Source: three-view drawing plus pictorial views. Frame: mm from the lowest corner of the part. A direction names the side the tool comes from. Give positions to 0.01 mm unless a question says otherwise; leave off trailing zeros. Write each loop counter-clockwise with the first axis right and the second up, starting at its lowest first coordinate (ties: lowest second). Pieces come first, ordered by that corner, then holes.
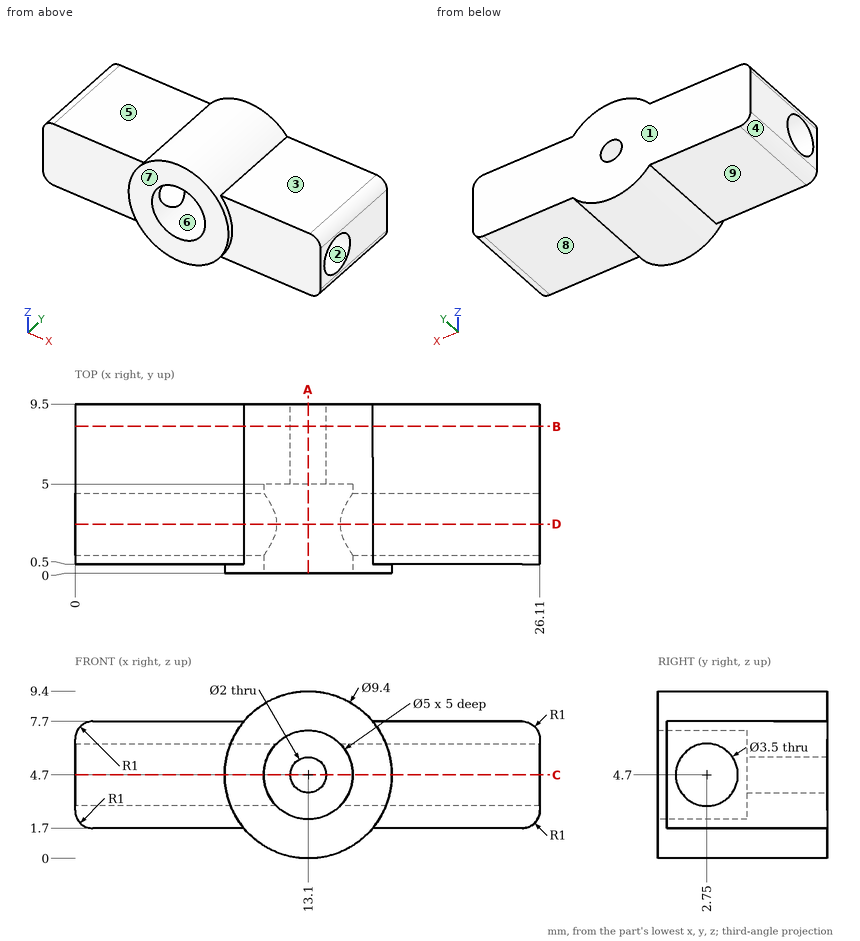
Q1. Section D-D on y = 2.75. Output: boundary loops of the cut face in (x, z), plus the area to 3 significant figures.
Filled sheet:
outline: (0, 2.7) arc R1 ccw to (1, 1.7) - (9.48, 1.7) arc R4.7 ccw to (16.72, 1.7) - (25.11, 1.7) arc R1 ccw to (26.11, 2.7) - (26.11, 2.95) - (14.89, 2.95) arc R2.5 cw to (11.31, 2.95) - (0, 2.95) - close; (0, 6.45) - (11.31, 6.45) arc R2.5 cw to (14.89, 6.45) - (26.11, 6.45) - (26.11, 6.7) arc R1 ccw to (25.11, 7.7) - (16.72, 7.7) arc R4.7 ccw to (9.48, 7.7) - (1, 7.7) arc R1 ccw to (0, 6.7) - close
area: 77.8 mm2
Q2. Ray query, line 1 along Y through (x, z) = (7, 4.7); line 2 along Y through (x, z) = (24.5, 2.5); line 3 along Z through (x, y) = (23.5, 7.5). Return the intervals inside material, ascending.
Filled sheet:
line 1: y = 0.5 to 1, 4.5 to 9.5
line 2: y = 0.5 to 9.5
line 3: z = 1.7 to 7.7
Q3. Pin query (flat end, axial travel): P1, Ø1.8, axis at x = 13.1, z = 4.7, coming from the +Y side; P2, Ø4, axis at x = 23, y = 3, coming from the +Z side; P3, Ø2.5, axis at x = 13, z = 4, coming from the -Y side; P4, Ø1.8, axis at x = 3.5, z = 5.5, coming from the -Y side. Return the tip coordinate at first contact, or that it passes through.
Filled sheet:
P1: passes through
P2: stops at z = 7.7
P3: stops at y = 5
P4: stops at y = 0.5
Q4. Section C-C on z = 4.7. Output: boundary loops of the cut face in (x, y).
Filled sheet:
outline: (0, 0.5) - (8.4, 0.5) - (8.4, 0) - (10.6, 0) - (10.6, 1) - (0, 1) - close; (0, 4.5) - (10.6, 4.5) - (10.6, 5) - (12.1, 5) - (12.1, 9.5) - (0, 9.5) - close; (14.1, 5) - (15.6, 5) - (15.6, 4.5) - (26.11, 4.5) - (26.11, 9.5) - (14.1, 9.5) - close; (15.6, 0) - (17.8, 0) - (17.8, 0.5) - (26.11, 0.5) - (26.11, 1) - (15.6, 1) - close
Q5. Section B-B on y = 8.25. Output: boundary loops of the cut face in (x, z).
Filled sheet:
outline: (0, 2.7) arc R1 ccw to (1, 1.7) - (9.48, 1.7) arc R4.7 ccw to (16.72, 1.7) - (25.11, 1.7) arc R1 ccw to (26.11, 2.7) - (26.11, 6.7) arc R1 ccw to (25.11, 7.7) - (16.72, 7.7) arc R4.7 ccw to (9.48, 7.7) - (1, 7.7) arc R1 ccw to (0, 6.7) - close; hole circle Ø2 at (13.1, 4.7)
Q6. Access query for the marked faces 5, 6, 7, 8 and 9. Directions: +Z, -Z, +X, -X, +Y, -Y. A direction counts if a zero-diameter tool reaches every point of the face in a straight line with its end or side. Return the directions, or none.
Filled sheet:
face 5: +Z, -X, +Y, -Y
face 6: -Y
face 7: +Z, -Z, +X, -X, -Y
face 8: -Z, +X, +Y, -Y
face 9: -Z, -X, +Y, -Y
Q7. Section A-A on x = 13.1. Output: boundary loops of the cut face in (y, z).
Filled sheet:
outline: (0, 0) - (9.5, 0) - (9.5, 3.7) - (5, 3.7) - (5, 2.2) - (0, 2.2) - close; (0, 7.2) - (5, 7.2) - (5, 5.7) - (9.5, 5.7) - (9.5, 9.4) - (0, 9.4) - close
Q8. Pull-direction query (Z, two-part tool) for the marked faces 1, 2, 3 and 4; classes: released by +Z, released by -Z, zero draft, split by the parting line, or undercut.
Filled sheet:
face 1: zero draft
face 2: undercut
face 3: released by +Z
face 4: released by -Z
